Print and shaded views of the part. All mm, measured from the part's lowest x, y and z. Round coordinates to 2 decimals unless told otherwise and drop trailing zeros. Order: outer loops, then holes, each group sorted by start corner. A loop starts at its lowest first (then second) coordinate and runs counter-clockwise, first axis right, second up. Notation, with made-up numbers: (25, -21) - (64, -21) arc R26 ccw to (64, 8) - close; hole circle Ø3 at (75, 25). An arc over 180 degrees is marked (long way). Return JSON: item names as keys, results as strings. Group by question number.
Item 1: Probe probe 1 along Z at (x, y) = (18, 92); probe 2 along X at (y, z) = (28.5, 115); probe 3 along X at (y, z) = (113, 115) (1 decimal). List the from-to ranges inside material, lowest first.
Item 2: Saw through at B-B on x = 60. List the corners of the cut face in (y, z) (1 decimal).
Item 3: Saw through at A-A on y = 48. List the corners of the cut face in (x, z).
Item 4: Drop flat-ended pins along their axis: pin 1 (5 mm diameter, centred on y = 30, z = 51, fed in from -X); pin 2 (10 mm diameter, centred on y = 21, z = 117.5, fed in from +X); pin 3 (2.5 mm diameter, centred on y = 15.5, z = 116, fed in from -X). Give the stop position or say it passes through.
Item 5: Saw through at C-C on y = 66. List the corners of the cut face in (x, z).
Item 6: Saw through at D-D on z = 10. List the corners of the cut face in (x, y) (1 decimal).
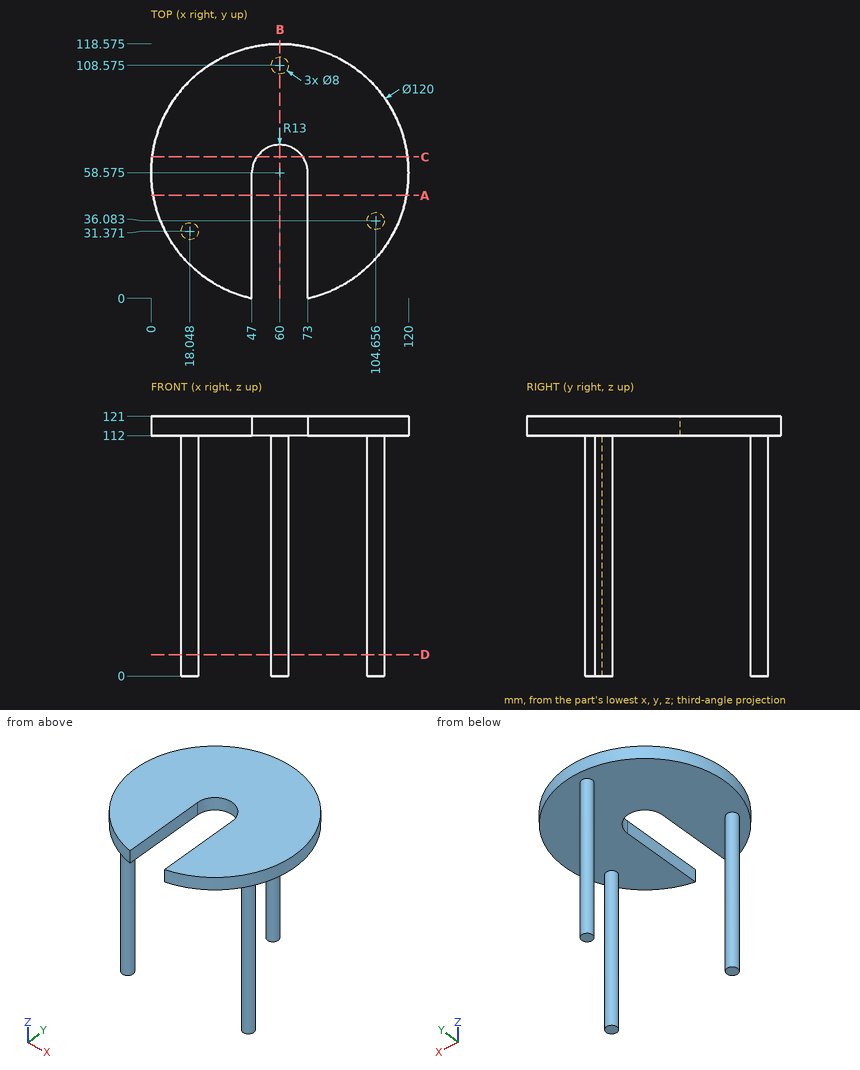
Filled in:
{
 "1": {"probe 1": "z = 112 to 121", "probe 2": "x = 8.08 to 47, 73 to 111.92", "probe 3": "x = 34.7 to 85.3"},
 "2": {"outline": "(71.6, 112) - (104.6, 112) - (104.6, 0) - (112.6, 0) - (112.6, 112) - (118.6, 112) - (118.6, 121) - (71.6, 121) - close"},
 "3": {"outline": "(0.94, 112) - (47, 112) - (47, 121) - (0.94, 121) - close; (73, 112) - (119.06, 112) - (119.06, 121) - (73, 121) - close"},
 "4": {"pin 1": "stops at x = 14.05", "pin 2": "stops at x = 110.39", "pin 3": "stops at x = 16.98"},
 "5": {"outline": "(0.46, 112) - (49.33, 112) - (49.33, 121) - (0.46, 121) - close; (70.67, 112) - (119.54, 112) - (119.54, 121) - (70.67, 121) - close"},
 "6": {"outline": "circle Ø8 at (18, 31.4); circle Ø8 at (60, 108.6); circle Ø8 at (104.7, 36.1)"}
}
